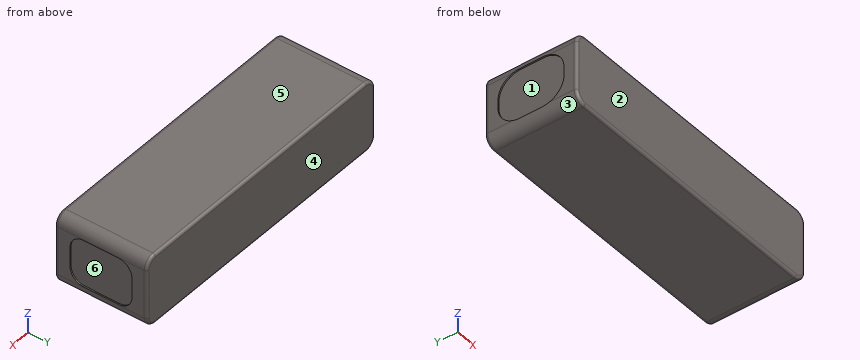
```python
from build123d import *

# Parameters (mm, degrees)
SKETCH1_W           = 107
SKETCH1_H           = 34
BOSS_EXTRUDE1_DEPTH = 26
CUT_EXTRUDE1_DEPTH  = 0.5
CUT_EXTRUDE2_DEPTH  = 0.5
FILLET1_R           = 4
FILLET2_R           = 1


with BuildPart() as part:
    # Sketch1 → Boss-Extrude1 (new body)
    with BuildSketch(Plane(origin=(0, 0, -15), x_dir=(-1, 0, 0), z_dir=(0, 0, -1))):
        with Locations((-15.5, -5)):
            Rectangle(SKETCH1_W, SKETCH1_H)
    extrude(amount=-BOSS_EXTRUDE1_DEPTH)

    # Sketch2 → Cut-Extrude1 (cut)
    with BuildSketch(Plane(origin=(69, 0, 0), x_dir=(0, 0, -1), z_dir=(1, 0, 0))):
        with BuildLine():
            Line((-6.75, 1.442307692), (-6.75, -11.442307692))
            ThreePointArc((-6.75, -11.442307692), (-5.285533906, -14.977841598), (-1.75, -16.442307692))
            Line((-1.75, -16.442307692), (5.75, -16.442307692))
            ThreePointArc((5.75, -16.442307692), (9.285533906, -14.977841598), (10.75, -11.442307692))
            Line((10.75, -11.442307692), (10.75, 1.442307692))
            ThreePointArc((10.75, 1.442307692), (9.285533906, 4.977841598), (5.75, 6.442307692))
            Line((5.75, 6.442307692), (-1.75, 6.442307692))
            ThreePointArc((-1.75, 6.442307692), (-5.285533906, 4.977841598), (-6.75, 1.442307692))
        make_face()
    extrude(amount=-CUT_EXTRUDE1_DEPTH, mode=Mode.SUBTRACT)

    # Sketch3 → Cut-Extrude2 (cut)
    with BuildSketch(Plane.ZY.offset(38)):
        with BuildLine():
            Line((-0.625, 7.259615385), (-3.375, 7.259615385))
            ThreePointArc((-3.375, 7.259615385), (-9.031854249, 4.916469634), (-11.375, -0.740384615))
            Line((-11.375, -0.740384615), (-11.375, -9.259615385))
            ThreePointArc((-11.375, -9.259615385), (-9.031854249, -14.916469634), (-3.375, -17.259615385))
            Line((-3.375, -17.259615385), (-0.625, -17.259615385))
            ThreePointArc((-0.625, -17.259615385), (5.031854249, -14.916469634), (7.375, -9.259615385))
            Line((7.375, -9.259615385), (7.375, -0.740384615))
            ThreePointArc((7.375, -0.740384615), (5.031854249, 4.916469634), (-0.625, 7.259615385))
        make_face()
    extrude(amount=-CUT_EXTRUDE2_DEPTH, mode=Mode.SUBTRACT)

    # Fillet1
    # the kernel refuses this fillet: 4 mm, written as the material it takes off along each edge
    with BuildSketch(Plane(origin=(-38, -32, -15), x_dir=(0, 0, 1), z_dir=(0, 1, 0)), Plane(origin=(69, 22, -15), x_dir=(0, 0, 1), z_dir=(0, -1, 0))) as fillet1_piece_1:
        with BuildLine():
            CenterArc((FILLET1_R, FILLET1_R), FILLET1_R, 180, 90)
            Line((0, FILLET1_R), (0, 0))
            Line((0, 0), (FILLET1_R, 0))
        make_face()
    extrude(amount=54, mode=Mode.SUBTRACT)
    with BuildSketch(Plane(origin=(-38, -32, 11), x_dir=(0, 0, -1), z_dir=(0, 1, 0)), Plane(origin=(69, 22, 11), x_dir=(0, 0, -1), z_dir=(0, -1, 0))) as fillet1_piece_2:
        with BuildLine():
            CenterArc((FILLET1_R, -FILLET1_R), FILLET1_R, 90, 90)
            Line((0, -FILLET1_R), (0, 0))
            Line((0, 0), (FILLET1_R, 0))
        make_face()
    extrude(amount=54, mode=Mode.SUBTRACT)

    # Fillet2
    fillet2_edges = [part.edges().sort_by_distance(p)[0] for p in [
        (15.5, -22, -15),
        (15.5, 12, -15),
        (-38, 12, -2),
        (15.5, 12, 11),
        (69, 12, -2),
        (67.828427125, 12, 9.828427125),
        (67.828427125, 12, -13.828427125),
        (-36.828427125, 12, 9.828427125),
        (-36.828427125, 12, -13.828427125),
        (-38, -22, -2),
        (69, -22, -2),
        (15.5, -22, 11),
        (67.828427125, -22, 9.828427125),
        (67.828427125, -22, -13.828427125),
        (-36.828427125, -22, 9.828427125),
        (-36.828427125, -22, -13.828427125),
    ]]
    fillet(fillet2_edges, radius=FILLET2_R)


solid = part.part
```
Geometry check sheet. Reference: the model listing, model coordinates, mm. Face numbers are marked on the shaded views. A direction names the side the tool comes from. Coordinates: 2 decimals unless noted, no trailing zeros. Use one line per item in the form item = value.
1. Scan lines: line 1 (X direction, y = -7.5, z = 5.25); line 2 (Z direction, x = 51, y = 11.5); line 3 (X direction, y = 6.5, z = 8.75). Record each from-to range of solid material in increasing order.
Here are the results:
line_1 = -37.5 to 68.5
line_2 = -14.87 to 10.87
line_3 = -37.6 to 68.6
2. Gauge pin test, flat ends, axial feed: pin 1 (0.6 mm diameter, centred on x = 68.5, z = -2, fed in from -Y); pin 2 (1.5 mm diameter, centred on y = -3.5, z = -3.5, fed in from +X); pin 3 (9.5 mm diameter, centred on y = -8.5, z = 1.5, fed in from -X). Record the tip position at first contact, or that the pin passes through.
Here are the results:
pin_1 = -21.98
pin_2 = 68.5
pin_3 = -37.5
3. Access from +Z, -Z, +X, -X, +Y, -Y to the whole of each face (thin tool, end or side, straight path). Record for the marked faces 1 and 2.
Here are the results:
face_1 = -X
face_2 = +Z, -Z, +X, -X, -Y
4. Draft check along Z on the marked faces 3, 4, 5 and 6. Enter one of: pulls with the +Z half, pulls with the -Z half, needs draft (parallel to the pull), parting line crosses it, or undercut.
Here are the results:
face_3 = pulls with the -Z half
face_4 = needs draft
face_5 = pulls with the +Z half
face_6 = undercut
